The listing builds one solid part. Answer for the finished solid, in the listing's coordinates (mm). A direction names the side the tool comes from. Coordinates: 2 decimals unless noted, no trailing zeros. Write each loop counter-clockwise with the first axis right and the second up, starting at its lowest first coordinate (ties: lowest second). Pieces come first, ordered by that corner, then holes.
from build123d import *

# Parameters (mm, degrees)
SCHIZZO1_R                   = 9.5
SCHIZZO1_R_2                 = 7
ESTRUSIONE_ESTRUSIONE2_DEPTH = 15.5
SCHIZZO2_R                   = 7
SCHIZZO2_R_2                 = 4.5
ESTRUSIONE_ESTRUSIONE3_DEPTH = 14.9
SMUSSO1_SIZE                 = 0.35


with BuildPart() as part:
    # Schizzo1 → Estrusione-Estrusione2 (new body)
    with BuildSketch(Plane.XY):
        Circle(SCHIZZO1_R)
        Circle(SCHIZZO1_R_2, mode=Mode.SUBTRACT)
    extrude(amount=ESTRUSIONE_ESTRUSIONE2_DEPTH)

    # Schizzo2 → Estrusione-Estrusione3 (add)
    with BuildSketch(Plane(origin=(0, 0, 0.3), x_dir=(-1, 0, 0), z_dir=(0, 0, -1))):
        Circle(SCHIZZO2_R)
        Circle(SCHIZZO2_R_2, mode=Mode.SUBTRACT)
    extrude(amount=-ESTRUSIONE_ESTRUSIONE3_DEPTH)

    # Smusso1
    smusso1_edges = [part.edges().sort_by_distance(p)[0] for p in [
        (-9.5, 0, 0),
        (-9.5, 0, 15.5),
    ]]
    chamfer(smusso1_edges, length=SMUSSO1_SIZE)


solid = part.part
1. For a pull along X with two mould halves and no side action, classify faces 3 (the cylindrical face through (4.38, -8.43, 7.65)), 4 (the flat face through (-2, -7, 0)), 5 (the flat face through (0, -5, 0.3)) as pulls with the +X half, pulls with the -X half, needs draft (parallel to the pull), parting line crosses it, or undercut.
Results found:
face 3: parting line crosses it
face 4: needs draft
face 5: undercut
2. A tool of negligible diameter and unlimited length cuts with its end or side. For faces 1 (the flat face through (0, -5, 15.2)), 2 (the flat face through (-2, -7, 15.5)), from which of +Z, -Z, +X, -X, +Y, -Y can it reach the whole face along a straight path? Write none if from no direction.
Results found:
face 1: +Z
face 2: +Z, +X, -X, +Y, -Y
3. Find the intervals of material crossed by L1, parallel to Y at x = 0, z = 11; L2, parallel to Y at x = 2, z = 12; L3, parallel to Z at x = 3.75, y = 2.75, in increasing order.
Results found:
L1: y = -9.5 to -4.5, 4.5 to 9.5
L2: y = -9.29 to -4.03, 4.03 to 9.29
L3: z = 0.3 to 15.2
4. Section A-A on y = 0 is taken. Give the vertices of the cut face in (x, z).
Results found:
outline: (-9.5, 0.35) - (-9.15, 0) - (-7, 0) - (-7, 0.3) - (-4.5, 0.3) - (-4.5, 15.2) - (-7, 15.2) - (-7, 15.5) - (-9.15, 15.5) - (-9.5, 15.15) - close; (4.5, 0.3) - (7, 0.3) - (7, 0) - (9.15, 0) - (9.5, 0.35) - (9.5, 15.15) - (9.15, 15.5) - (7, 15.5) - (7, 15.2) - (4.5, 15.2) - close
5. Section C-C on z = 4.5 is taken. Give the vertices of the cut face in (x, y), then the cut area to 3 significant figures.
Results found:
outline: circle Ø19 at (0, 0); hole circle Ø9 at (0, 0)
area: 220 mm2
6. Flat-ended cylindrical pins translate along their axes: P1, Ø7, axis at x = 0, y = 0, coming from the +Z side; P2, Ø11, axis at x = 3.5, y = -3, coming from the +Z side; P3, Ø6, axis at x = 1.5, y = -3.5, coming from the +Z side; P4, Ø5, axis at y = -5.5, z = 12, coming from the +X side. Find the tip coordinate at first contact, or state that the pin passes through.
Results found:
P1: passes through
P2: stops at z = 15.5
P3: stops at z = 15.2
P4: stops at x = 9.01
